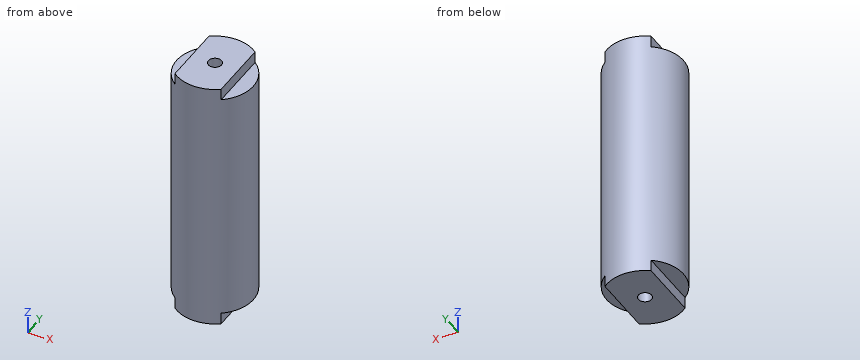
```python
from build123d import *

# Parameters (mm, degrees)
SKETCH1_R           = 26.3525
BOSS_EXTRUDE1_DEPTH = 88.9
CUT_EXTRUDE1_DEPTH  = 7.9502
CUT_EXTRUDE2_START  = -3
SKETCH3_R           = 22.86
CUT_EXTRUDE2_DEPTH  = 155.8996
SKETCH5_R           = 4.5
CUT_EXTRUDE3_DEPTH  = 182.663833804


with BuildPart() as part:
    # Sketch1 → Boss-Extrude1 (new, symmetric)
    with BuildSketch(Plane.XY):
        Circle(SKETCH1_R)
    extrude(amount=BOSS_EXTRUDE1_DEPTH, both=True)

    # Sketch2 → Cut-Extrude1 (cut)
    with BuildSketch(Plane.XY.offset(88.9)):
        with BuildLine():
            Line((-15.875, 21.034225235), (-15.875, -21.034225235))
            ThreePointArc((-15.875, -21.034225235), (-26.3525, 0), (-15.875, 21.034225235))
        make_face()
        with BuildLine():
            Line((15.875, -21.034225235), (15.875, 21.034225235))
            ThreePointArc((15.875, 21.034225235), (26.3525, 0), (15.875, -21.034225235))
        make_face()
    cut_extrude1 = extrude(amount=-CUT_EXTRUDE1_DEPTH, mode=Mode.SUBTRACT)

    # Mirror1: Cut-Extrude1 across plane
    add(cut_extrude1.mirror(Plane.XY), mode=Mode.SUBTRACT)

    # Sketch3 → Cut-Extrude2 (cut)
    with BuildSketch(Plane.XY.offset(80.9498).offset(CUT_EXTRUDE2_START)):
        Circle(SKETCH3_R)
    extrude(amount=-CUT_EXTRUDE2_DEPTH, mode=Mode.SUBTRACT)

    # Sketch5 → Cut-Extrude3 (cut, through all)
    with BuildSketch(Plane.XY.offset(88.9)):
        Circle(SKETCH5_R)
    extrude(amount=-CUT_EXTRUDE3_DEPTH, mode=Mode.SUBTRACT)


solid = part.part
```
Source: CAD feature listing. Evaluate the final solid. Frame: model axes, mm. Round coordinates to 2 decimals unless told otherwise and drop trailing zeros. Order: outer loops, then holes, each group sorted by start corner. A loop starts at its lowest first (then second) coordinate and runs counter-clockwise, first axis right, second up. Notation, with made-up numbers: (51.25, 68.5) -> (55.25, 68.5) arc R31 cw to (55.25, 92.5) -> close; hole circle Ø11 at (16, 87.25). An arc over 180 degrees is marked (long way). One line per item, written item: value. Start each with the question number.
Q1. Section query C-C (z = 58.5). Return the cut outline in (x, y) (1 decimal), plus the area to 3 significant figures.
Q2. Pin query (flat end, axial travel): pin 1 (1 mm diameter, centred on y = -5.5, z = 7, fed in from -X); pin 2 (2.5 mm diameter, centred on y = -1.5, z = 83, fed in from -X) (3 decimals); pin 3 (8.5 mm diameter, centred on y = 0, z = -87, fed in from +X) (3 decimals). Return the tip coordinate at first contact, or that it passes through.
Q3. Material intervals for probe 1 along Z at (x, y) = (-3, 21); probe 2 along Y at (x, z) = (-17, 54); probe 3 along X at (y, z) = (7, 28), sorted ascending.
Q4. Section query B-B (x = 0). Return the cut outline in (y, z), plus the area to 3 significant figures.
Q5. Section query A-A (y = 0). Return the cut outline in (x, z) (1 decimal), plus the area to 3 significant figures.
Q6. Section query D-D (x = -17.5). Return the cut outline in (y, z), plus the area to 3 significant figures.
Findings below:
1. outline: circle Ø52.7 at (0, 0); hole circle Ø45.7 at (0, 0)
1. area: 540 mm²
2. pin 1: x = -25.87
2. pin 2: x = -15.875
2. pin 3: x = 15.875
3. probe 1: -88.9 to -77.95, 77.95 to 88.9
3. probe 2: -20.14 to -15.28, 15.28 to 20.14
3. probe 3: -25.41 to -21.76, 21.76 to 25.41
4. outline: (-26.35, -88.9) -> (-4.5, -88.9) -> (-4.5, -77.95) -> (-22.86, -77.95) -> (-22.86, 77.95) -> (-4.5, 77.95) -> (-4.5, 88.9) -> (-26.35, 88.9) -> close; (4.5, -88.9) -> (26.35, -88.9) -> (26.35, 88.9) -> (4.5, 88.9) -> (4.5, 77.95) -> (22.86, 77.95) -> (22.86, -77.95) -> (4.5, -77.95) -> close
4. area: 2,050 mm²
5. outline: (-26.4, -80.9) -> (-15.9, -80.9) -> (-15.9, -88.9) -> (-4.5, -88.9) -> (-4.5, -77.9) -> (-22.9, -77.9) -> (-22.9, 77.9) -> (-4.5, 77.9) -> (-4.5, 88.9) -> (-15.9, 88.9) -> (-15.9, 80.9) -> (-26.4, 80.9) -> close; (4.5, -88.9) -> (15.9, -88.9) -> (15.9, -80.9) -> (26.4, -80.9) -> (26.4, 80.9) -> (15.9, 80.9) -> (15.9, 88.9) -> (4.5, 88.9) -> (4.5, 77.9) -> (22.9, 77.9) -> (22.9, -77.9) -> (4.5, -77.9) -> close
5. area: 1,710 mm²
6. outline: (-19.7, -80.95) -> (19.7, -80.95) -> (19.7, 80.95) -> (-19.7, 80.95) -> close; hole (-14.71, -77.95) -> (14.71, -77.95) -> (14.71, 77.95) -> (-14.71, 77.95) -> close
6. area: 1,790 mm²
